Geometry: final body of the model. Coordinates: model frame, mm. Face numbers are marked on the shaded views. Give positions to 0.01 mm unless a question says otherwise; leave off trailing zeros. Write each loop counter-clockwise with the first axis right and the second up, starting at its lowest first coordinate (ties: lowest second). Pieces come first, ordered by that corner, then holes. Notation, with made-up numbers: (2, -25) -> (24, -25) arc R25 cw to (24, -11) -> close; hole circle Ø7 at (57.25, -39.75). An arc over 180 degrees is marked (long way). Answer in a Markdown table with one row per item. Add a question column.
Item 1: Section query A-A on x = 0. Output: boundary loops of the cut face in (y, z) (3 decimals), plus the area to 4 significant figures.
Item 2: Section query B-B on z = 2.35. Output: boundary loops of the cut face in (x, y) (3 decimals), plus the area to 3 significant figures.
Item 3: First-contact query: P1, Ø2, axis at x = -9.5, y = 13.5, coming from the -Z side. Flat tip, straight axial feed; report the tip coordinate or a pass-through.
Item 4: Draft query along X for the marked faces 1, 2, 3 and 4. Return one class per face: +X half, -X half, draft (parallel to the pull), parting line (faces both ways), or undercut.
Item 5: Material intervals for probe 1 along Y at (x, z) = (6.35, 1.15); probe 2 along Y at (x, z) = (0, 0.8); probe 3 along X at (y, z) = (-1.5, 2.5), sorted ascending. Write a range as from..to.
Item 6: Section query C-C on x = 8. Output: boundary loops of the cut face in (y, z) (3 decimals), plus the area to 3 significant figures.
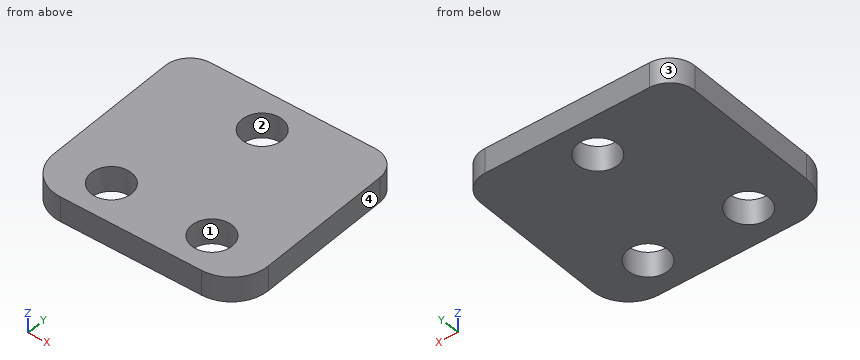
```python
from build123d import *

# Parameters (mm, degrees)
BOSS_EXTRUDE1_DEPTH    = 3.175
F_10_CLEARANCE_HOLE1_D = 5.1054


with BuildPart() as part:
    # Sketch1 → Boss-Extrude1 (new body)
    with BuildSketch(Plane.XY):
        with BuildLine():
            Line((-8.9027, 4.6609), (8.9027, 4.6609))
            ThreePointArc((8.9027, 4.6609), (12.198453996, 3.295753996), (13.5636, 0))
            Line((13.5636, 0), (13.5636, 17.3482))
            ThreePointArc((13.5636, 17.3482), (12.63366403, 19.59326403), (10.3886, 20.5232))
            Line((10.3886, 20.5232), (-10.3886, 20.5232))
            ThreePointArc((-10.3886, 20.5232), (-12.63366403, 19.59326403), (-13.5636, 17.3482))
            Line((-13.5636, 17.3482), (-13.5636, 0))
            ThreePointArc((-13.5636, 0), (-12.198453996, 3.295753996), (-8.9027, 4.6609))
        make_face()
        with BuildLine():
            ThreePointArc((13.5636, 0), (12.198453996, 3.295753996), (8.9027, 4.6609))
            Line((8.9027, 4.6609), (-8.9027, 4.6609))
            ThreePointArc((-8.9027, 4.6609), (-12.198453996, 3.295753996), (-13.5636, 0))
            ThreePointArc((-13.5636, 0), (-12.198453996, -3.295753996), (-8.9027, -4.6609))
            Line((-8.9027, -4.6609), (8.9027, -4.6609))
            ThreePointArc((8.9027, -4.6609), (12.198453996, -3.295753996), (13.5636, 0))
        make_face()
    extrude(amount=BOSS_EXTRUDE1_DEPTH)

    # #10 Clearance Hole1 (through all)
    with Locations(Plane.XY.offset(3.175)):
        with Locations((6.35, 0.1016), (-6.35, 0.1016), (0, 15.7607)):
            Hole(F_10_CLEARANCE_HOLE1_D / 2)


solid = part.part
```
Findings below:
| question | item | result |
|---|---|---|
| 1 | outline | (-4.661, 0) -> (13.208, 0) -> (13.208, 3.175) -> (-4.661, 3.175) -> close; (18.313, 0) -> (20.523, 0) -> (20.523, 3.175) -> (18.313, 3.175) -> close |
| 1 | area | 63.75 mm^2 |
| 2 | outline | (-13.564, 0) arc R4.661 ccw to (-8.903, -4.661) -> (8.903, -4.661) arc R4.661 ccw to (13.564, 0) -> (13.564, 17.348) arc R3.175 ccw to (10.389, 20.523) -> (-10.389, 20.523) arc R3.175 ccw to (-13.564, 17.348) -> close; hole circle Ø5.105 at (-6.35, 0.102); hole circle Ø5.105 at (0, 15.761); hole circle Ø5.105 at (6.35, 0.102) |
| 2 | area | 608 mm^2 |
| 3 | P1 | stops at z = 0 |
| 4 | face 1 | undercut |
| 4 | face 2 | undercut |
| 4 | face 3 | -X half |
| 4 | face 4 | +X half |
| 5 | probe 1 | y = -4.66..-2.45, 2.65..20.52 |
| 5 | probe 2 | y = -4.66..13.21, 18.31..20.52 |
| 5 | probe 3 | x = -13.32..-8.34, -4.36..4.36, 8.34..13.32 |
| 6 | outline | (-4.661, 0) -> (-1.846, 0) -> (-1.846, 3.175) -> (-4.661, 3.175) -> close; (2.049, 0) -> (20.523, 0) -> (20.523, 3.175) -> (2.049, 3.175) -> close |
| 6 | area | 67.6 mm^2 |
